Print and shaded views of the part. All mm, measured from the part's lowest x, y and z. Round coordinates to 2 decimals unless told otherwise and drop trailing zeros. Loops run counter-clockwise (first coordinate to the right, second up) from the corner with the lowest first, then second, coordinate; pieces in that order, holes last. Notation, with made-up numbers: (1, -7.75) -> (30, -7.75) arc R23 ccw to (30, 21.25) -> close; hole circle Ø5 at (8.5, 21.25). An arc over 180 degrees is marked (long way). Use a Markdown table: item, result.
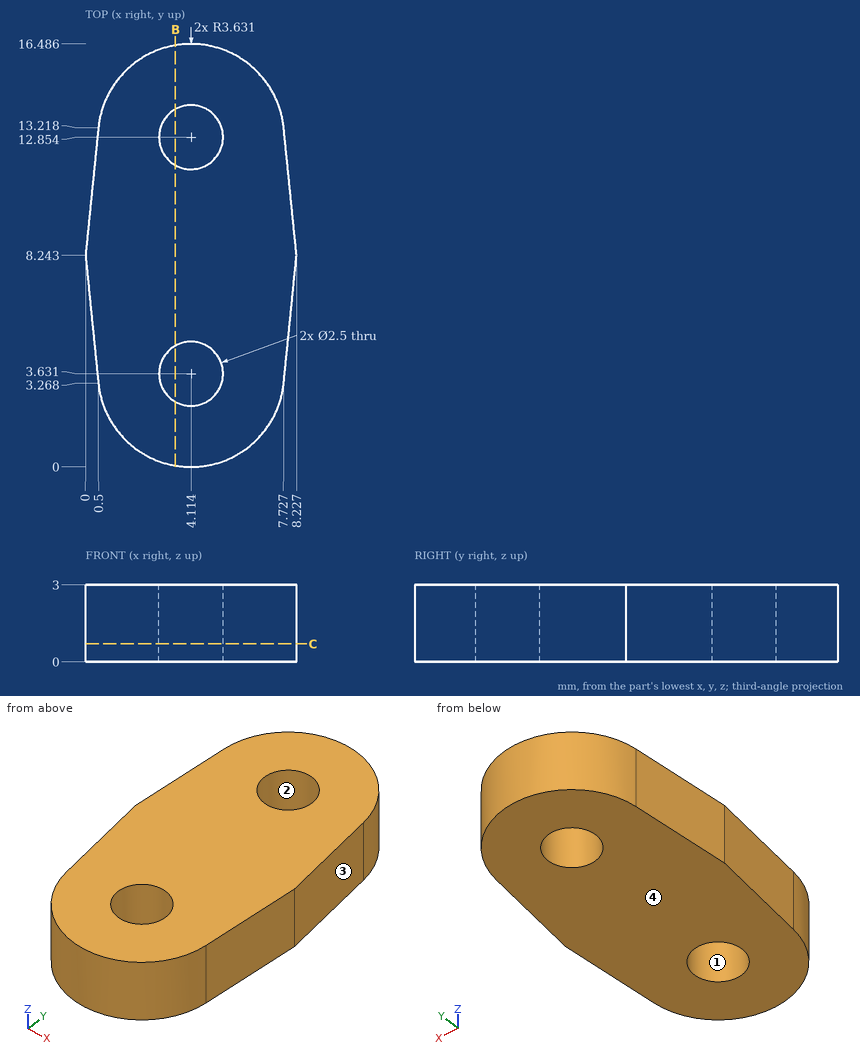
Q1. Flat gauge pins, fed straight in: pin 1 (1.5 mm diameter, centred on y = 7, z = 0.5, fed in from +X); pin 2 (1 mm diameter, centred on y = 6, z = 2.5, fed in from -X) (1 decimal); pin 3 (1.5 mm diameter, centred on y = 9.5, z = 2.5, fed in from -X). Where does each tip first touch, or does it go through?
Results list:
| item | result |
|---|---|
| pin 1 | stops at x = 8.18 |
| pin 2 | stops at x = 0.2 |
| pin 3 | stops at x = 0.05 |
Q2. Pull direction Y, two halves, no side cores. Call the marked faces 1, 2, 3 and 4: released by +Y, released by -Y, zero draft, split by the parting line, or undercut.
Results list:
| item | result |
|---|---|
| face 1 | undercut |
| face 2 | undercut |
| face 3 | released by +Y |
| face 4 | zero draft |
Q3. Band-saw the part on C-C, the plane z = 0.7. Give the number of separate pieces and of enclosed holes in the cut face, plus the area to 3 significant figures.
Results list:
| item | result |
|---|---|
| separate pieces | 1 |
| enclosed holes | 2 |
| area | 103 mm² |
Q4. Band-saw the part on B-B, the plane x = 3.5. Give the cut face in (y, z) (1 decimal).
Results list:
| item | result |
|---|---|
| outline | (0.1, 0) -> (2.5, 0) -> (2.5, 3) -> (0.1, 3) -> close; (4.7, 0) -> (11.8, 0) -> (11.8, 3) -> (4.7, 3) -> close; (13.9, 0) -> (16.4, 0) -> (16.4, 3) -> (13.9, 3) -> close |
Q5. Drill centre lines: L1, parallel to Y at x = 4.5, z = 0.9 (1 decimal); L2, parallel to X at y = 4, z = 2.45; L3, parallel to Y at x = 3, z = 0.2 (1 decimal). Where is each one in solid material? Low to high. Write a range as from..to.
Results list:
| item | result |
|---|---|
| L1 | y = 0..2.4, 4.8..11.7, 14..16.5 |
| L2 | x = 0.43..2.92, 5.31..7.8 |
| L3 | y = 0.2..3.1, 4.2..12.3, 13.4..16.3 |
